Autodesk Inventor part; units mm, degrees
ref_plane "YZ Plane" through (0, 0, 0) normal (1, 0, 0) x (0, 1, 0)
ref_plane "XZ Plane" through (0, 0, 0) normal (0, 1, 0) x (-1, 0, 0)
ref_plane "XY Plane" through (0, 0, 0) normal (0, 0, 1) x (1, 0, 0)
sketch "Sketch1" plane through (0, 0, 0) normal (0, 0, 1) x (1, 0, 0)
  circle A0 centre (0, 0) radius 26.1874
  circle A1 centre (0, 0) radius 23.6474
  dimension "d0" = 52.3748
  dimension "d1" = 2.54
extrude "Extrusion1" add sketch "Sketch1" along normal mid plane 272.288
sketch "Sketch2" plane through (0, 0, 0) normal (1, 0, 0) x (0, 1, 0)
  line L0 (-26.1874, 136.144) -> (26.1874, 136.144)
  line L1 (-23.6474, 136.144) -> (23.6474, 136.144)
  line L2 (26.1874, 136.144) -> (25.4, 136.144)
  line L3 (25.4, 136.144) -> (25.4, 134.5565)
  line L4 (25.4, 134.5565) -> (26.1874, 134.5565)
  line L5 (26.1874, 134.5565) -> (26.1874, 136.144)
  line L6 (0, -14.5288) -> (0, 87.1728)
  point P0 (0, 0)
  dimension "d4" = 1.5875
  dimension "d5" = 0.7874
revolve "Revolution1" cut sketch "Sketch2" angle 360 about axis through (0, 0, -10) along (0, 0, 1)
mirror "Mirror1" about plane through (0, 0, 0) normal (0, 0, 1) of "Revolution1"
properties part number "AVT-32-32_Body Tube" material "Stainless Steel"
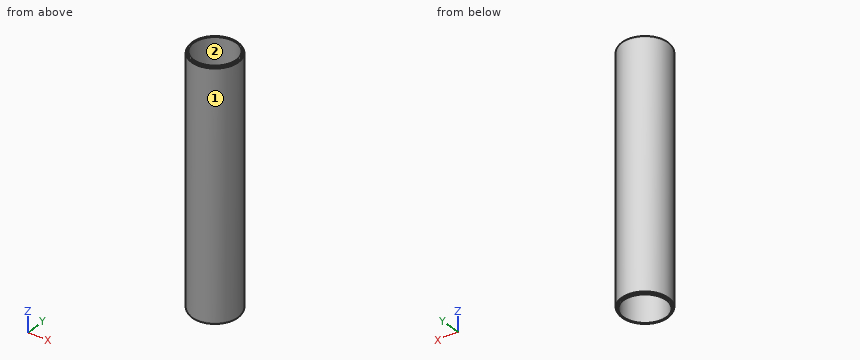
For this review, take the finished solid that the model builds, in its own axes (mm). Face numbers are marked on the shaded views. Round coordinates to 2 decimals unless told otherwise and drop trailing zeros. Write each loop counter-clockwise with the first axis right and the second up, starting at its lowest first coordinate (ties: lowest second). Pieces come first, ordered by that corner, then holes. Notation, with made-up numbers: (40, 77.5) - (75, 77.5) arc R32 cw to (75, 114.5) - close; hole circle Ø3 at (81.25, 5). An arc over 180 degrees is marked (long way). Write item = value, one per line. Start each with the question number.
1. Draft analysis for pull direction X (two halves, no side actions). For the marked faces 1 and 2, state which applies: released by +X, released by -X, zero draft, split by the parting line, or undercut.
2. Consider section A-A on x = 0. State the section outline as (y, z) points.
3. Consider section C-C on z = -33. State the section outline as (x, y) points.
4. Wall thickness on L1, parallel to Y at x = -1, z = 72; L2, parallel to X at y = -2.5, z = -110.5; L3, parallel to X at y = 21, z = -62: over which ranges is each line inside the solid? List them lowest first.
5. For pin 1 Ø10 at (x, z) = (-18, 26.5) entering from -Y; pin 2 Ø12 at (x, z) = (-13.5, 28) entering from -Y; pin 3 Ø10 at (x, z) = (17.5, -50.5) entering from +Y, all flat-tipped, find the tip position at first contact; note any pin that passes through.
Evaluation:
q1.face_1 = split by the parting line
q1.face_2 = undercut
q2.outline = (-26.19, -134.56) - (-25.4, -134.56) - (-25.4, -136.14) - (-23.65, -136.14) - (-23.65, 136.14) - (-25.4, 136.14) - (-25.4, 134.56) - (-26.19, 134.56) - close; (23.65, -136.14) - (25.4, -136.14) - (25.4, -134.56) - (26.19, -134.56) - (26.19, 134.56) - (25.4, 134.56) - (25.4, 136.14) - (23.65, 136.14) - close
q3.outline = circle Ø52.37 at (0, 0); hole circle Ø47.29 at (0, 0)
q4.L1 = -26.17 to -23.63, 23.63 to 26.17
q4.L2 = -26.07 to -23.51, 23.51 to 26.07
q4.L3 = -15.65 to -10.87, 10.87 to 15.65
q5.pin_1 = -22.73
q5.pin_2 = -25.09
q5.pin_3 = 23.01
